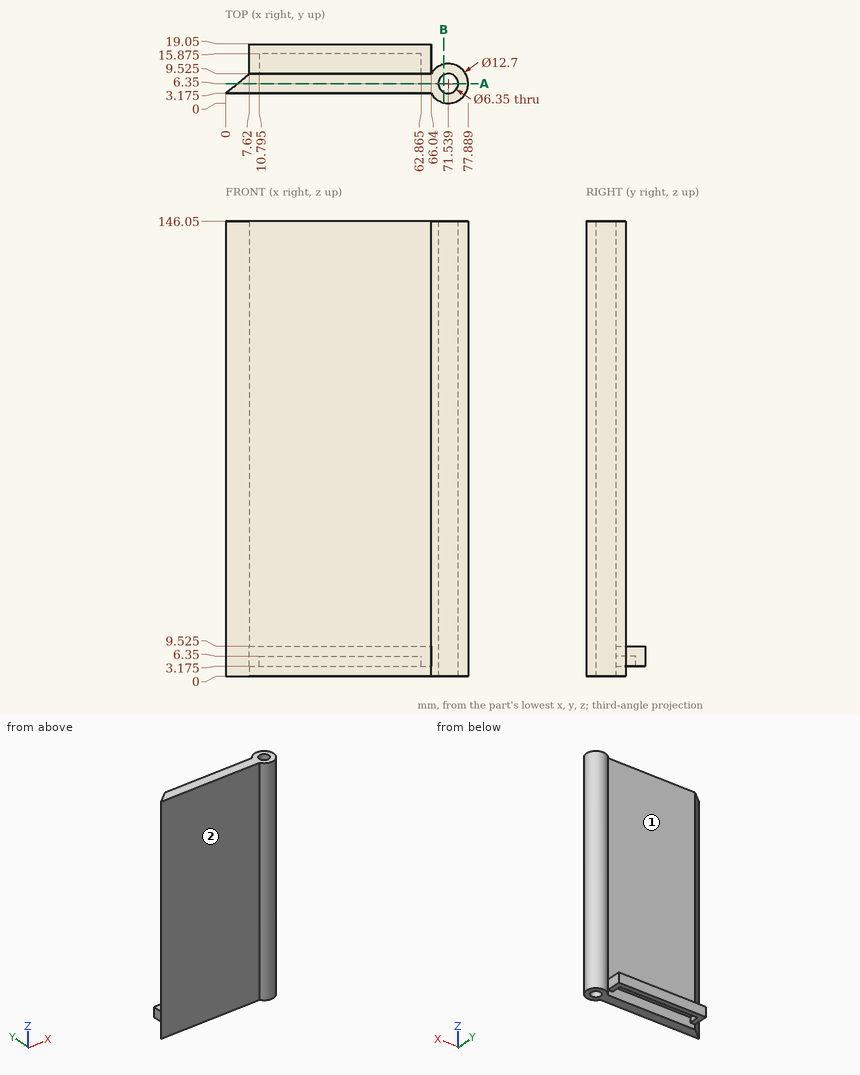
Answer from the drawing. Dimensions are ordinates in mm from the lowest x, y and z of the part. A direction names the side the tool comes from. Coordinates: 2 decimals unless noted, no trailing zeros. Write each loop counter-clockwise with the first axis right and the second up, starting at its lowest first coordinate (ties: lowest second). Pieces come first, ordered by that corner, then holes. Notation, with made-up numbers: M -3,84 L 17,84 A20 ccw 17,121 Z; hole C 73.25,-15 d5. An arc over 180 degrees is marked long. Put each result on its own line as item: value. Start each with the question number.
1. A cutting plane is placed at A-A on y = 6.35. Write down the section's boundary in (x, z), then the cut area to 3 significant figures.
2. Flat-ended cylindrical pins translate along their axes: P1, Ø3, axis at y = 12, z = 5, coming from the +X side (1 decimal); P2, Ø1.6, axis at y = 13.5, z = 4, coming from the -X side; P3, Ø1.6, axis at x = 42, z = 4.5, coming from the -Y side (3 decimals); P4, Ø10.5, axis at x = 28, y = 13.5, coming from the +Z side. Find the tip coordinate at first contact, or state that the pin passes through.
3. A cutting plane is placed at B-B on x = 70. Write down the section's boundary in (y, z).
4. Which of the six approach directions +Z, -Z, +X, -X, +Y, -Y give full straight-line access (tool end or side, diameter ignored) to the marked faces 1 and 2?
5. Consider line 1 (Z direction, x = 15.5, y = 17) (1 decimal); line 2 (X direction, y = 10.5, z = 7) (1 decimal). Determine where each line is inside the solid, lowest interval first. Write a range as from..to.
Resolved:
1. outline: M 3.81,0 L 68.36,0 L 68.36,146.05 L 3.81,146.05 Z; M 74.71,0 L 77.89,0 L 77.89,146.05 L 74.71,146.05 Z
1. area: 9,890 mm2
2. P1: stops at x = 76.3
2. P2: stops at x = 7.62
2. P3: stops at y = 3.175
2. P4: stops at z = 146.05
3. outline: M 0.19,0 L 3.57,0 L 3.57,146.05 L 0.19,146.05 Z; M 9.13,0 L 12.51,0 L 12.51,146.05 L 9.13,146.05 Z
4. face 1: +Z, -X, +Y
4. face 2: +Z, -Z, -X, -Y
5. line 1: z = 3.2..9.5
5. line 2: x = 7.6..66, 66.7..76.3
